Could you check a few things on this model? Use its own coordinates, in mm. Face numbers are marked on the shaded views. A direction names the side the tool comes from. Give positions to 0.01 mm unless a question says otherwise; leave off trailing zeros. Order: outer loops, then holes, each group sorted by start corner. A loop starts at its lowest first (then second) coordinate and runs counter-clockwise, first axis right, second up. Notation, with made-up numbers: (-14, 89.25) -> (3, 89.25) arc R15 cw to (3, 95.25) -> close; hole circle Ø9 at (14, 8.25). An arc over 180 degrees is marked (long way). Write each question's results on one line, items separated by ' | '.
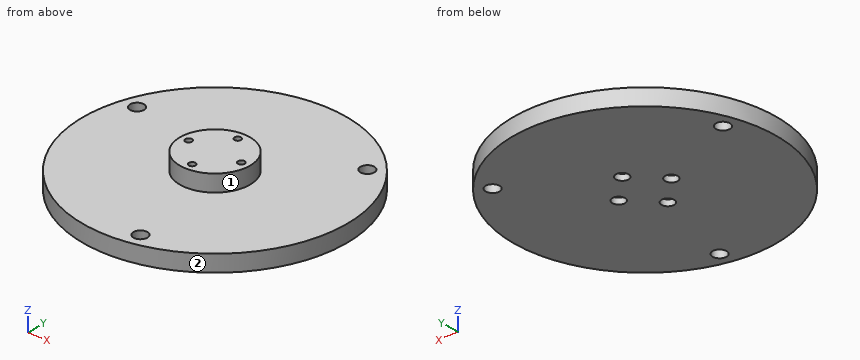
Autodesk Inventor part; units mm, degrees
ref_plane "YZ Plane" through (0, 0, 0) normal (1, 0, 0) x (0, 1, 0)
ref_plane "XZ Plane" through (0, 0, 0) normal (0, 1, 0) x (-1, 0, 0)
ref_plane "XY Plane" through (0, 0, 0) normal (0, 0, 1) x (1, 0, 0)
sketch "スケッチ1" plane through (0, 0, 0) normal (0, 0, 1) x (1, 0, 0)
  circle A0 centre (0, 0) radius 39.5
  circle A1 centre (26.1561, 23.2563) radius 2.1
  circle A2 centre (-33.2186, 11.0237) radius 2.1
  circle A3 centre (7.0625, -34.28) radius 2.1
  dimension "d0" = 79
  dimension "d3" = 4.2
  dimension "d4" = 35
  dimension "d7" = 360
extrude "押し出し1" add sketch "スケッチ1" along normal blind 5 contours A0 | A1 | A2 | A3
sketch "スケッチ2" plane through (0, 0, 5) normal (0, 0, 1) x (1, 0, 0)
  circle A0 centre (0, 0) radius 40
  circle A1 centre (26.1561, 23.2563) radius 2.1
  circle A2 centre (-33.2186, 11.0237) radius 2.1
  circle A3 centre (7.0625, -34.28) radius 2.1
  dimension "d11" = 80
  dimension "d12" = 4.2
  dimension "d13" = 35
  dimension "d14" = 360
extrude "押し出し2" cut sketch "スケッチ2" against normal blind 5 contours A1 | A2 | A3
sketch "スケッチ3" plane through (0, 0, 5) normal (0, 0, 1) x (1, 0, 0)
  circle A0 centre (0, 0) radius 10.5
  dimension "d17" = 21
extrude "押し出し3" add sketch "スケッチ3" along normal blind 5
sketch "スケッチ4" plane through (0, 0, 10) normal (0, 0, 1) x (1, 0, 0)
  circle A0 centre (0, 8) radius 1
  line L0 (0, -55.3) -> (0, 55.3)
  circle A1 centre (-8, 0) radius 1
  circle A2 centre (0, -8) radius 1
  circle A3 centre (8, 0) radius 1
  point P0 (0, 0)
  dimension "d20" = 2
  dimension "d21" = 8
  dimension "d24" = 360
extrude "押し出し4" cut sketch "スケッチ4" against normal blind 10
sketch "スケッチ5" plane through (0, 0, 0) normal (0, 0, -1) x (-1, 0, 0)
  circle A0 centre (-8, 0) radius 1
  circle A1 centre (-8, 0) radius 1.9
  circle A2 centre (0, -8) radius 1.9
  circle A3 centre (8, 0) radius 1.9
  circle A4 centre (0, 8) radius 1.9
  point P0 (0, 0)
  dimension "d28" = 3.8
  dimension "d31" = 360
extrude "押し出し5" cut sketch "スケッチ5" against normal blind 1.8
properties part number "rotate_plate_4"
Q1. Suppose I cut it at D-D on y = -34.28. Please give me the cut outline in (x, z), and give its area (3 significant figures).
Here are the results:
outline: (-19.62, 0) -> (4.96, 0) -> (4.96, 5) -> (-19.62, 5) -> close; (9.16, 0) -> (19.62, 0) -> (19.62, 5) -> (9.16, 5) -> close | area: 175 mm²
Q2. I'm going to push flat-ended pins straight in: pin 1 Ø3.5 at (x, y) = (26.16, 23.26) entering from -Z; pin 2 Ø2 at (y, z) = (8.5, 2) entering from -X; pin 3 Ø1 at (x, y) = (-17.5, 1.5) entering from +Z; pin 4 Ø2 at (x, z) = (23, 4.5) entering from +Y. Where does each tip first touch, or does it pass through?
Here are the results:
pin 1: passes through | pin 2: stops at x = -38.78 | pin 3: stops at z = 5 | pin 4: stops at y = 32.81
Q3. I need wall thicknesses on line 1 along Y through (x, z) = (0, 7.5); line 2 along Z through (x, y) = (-25.5, -19); line 3 along Y through (x, z) = (8, 5.25). Which ranges of each line are inside material? Lowest first, please.
Here are the results:
line 1: y = -10.5 to -9, -7 to 7, 9 to 10.5 | line 2: z = 0 to 5 | line 3: y = -6.8 to -1, 1 to 6.8
Q4. For the marked faces 1 and 2, which set-ups out of +Z, -Z, +X, -X, +Y, -Y let a thin tool reach every point of the face, with its end or its side?
Here are the results:
face 1: +Z | face 2: +Z, -Z
Q5. Suppose I cut it at A-A on x = 0. Please give me the cut outline in (y, z).
Here are the results:
outline: (-39.5, 0) -> (-9.9, 0) -> (-9.9, 1.8) -> (-9, 1.8) -> (-9, 10) -> (-10.5, 10) -> (-10.5, 5) -> (-39.5, 5) -> close; (-7, 1.8) -> (-6.1, 1.8) -> (-6.1, 0) -> (6.1, 0) -> (6.1, 1.8) -> (7, 1.8) -> (7, 10) -> (-7, 10) -> close; (9, 1.8) -> (9.9, 1.8) -> (9.9, 0) -> (39.5, 0) -> (39.5, 5) -> (10.5, 5) -> (10.5, 10) -> (9, 10) -> close
Q6. Suppose I cut it at C-C on z = 8.75. Please give me the cut outline in (x, y), and give its area (3 significant figures).
Here are the results:
outline: circle Ø21 at (0, 0); hole circle Ø2 at (-8, 0); hole circle Ø2 at (0, -8); hole circle Ø2 at (0, 8); hole circle Ø2 at (8, 0) | area: 334 mm²
